Job drawing, mm, ordinate dimensions from the low corner. One solid piece. Give positions to 0.01 mm unless a question says otherwise; leave off trailing zeros. Order: outer loops, then holes, each group sorted by start corner. A loop starts at its lowest first (then second) coordinate and runs counter-clockwise, first axis right, second up.
Item 1: Band-saw the part on B-B on x = 10. Give the cut face in (y, z), plus the area to 3 significant figures.
Item 2: Band-saw the part on C-C on z = 37.5. Give the cut face in (x, y), plus the area to 3 significant figures.
Item 3: Band-saw the part on A-A on y = 2.6. Give the cut face in (x, z).
Item 4: Two-plate mould, pull along Z, no slides. Class the marked faces 1 and 2: released by +Z, released by -Z, zero draft, split by the parting line, or undercut.
Item 5: Wall check: L1, parallel to X at y = 0.3, z = 37.5; L2, parallel to Z at x = 58.5, y = 2.55; L3, parallel to X at y = 2.25, z = 54. Give the ranges that are in metal, low to high.
Item 6: Flat gauge pin, fed straight in: P1, Ø6, axis at x = 16.5, z = 28, coming from the +Y side. Where does the tip first touch, or does it go through?
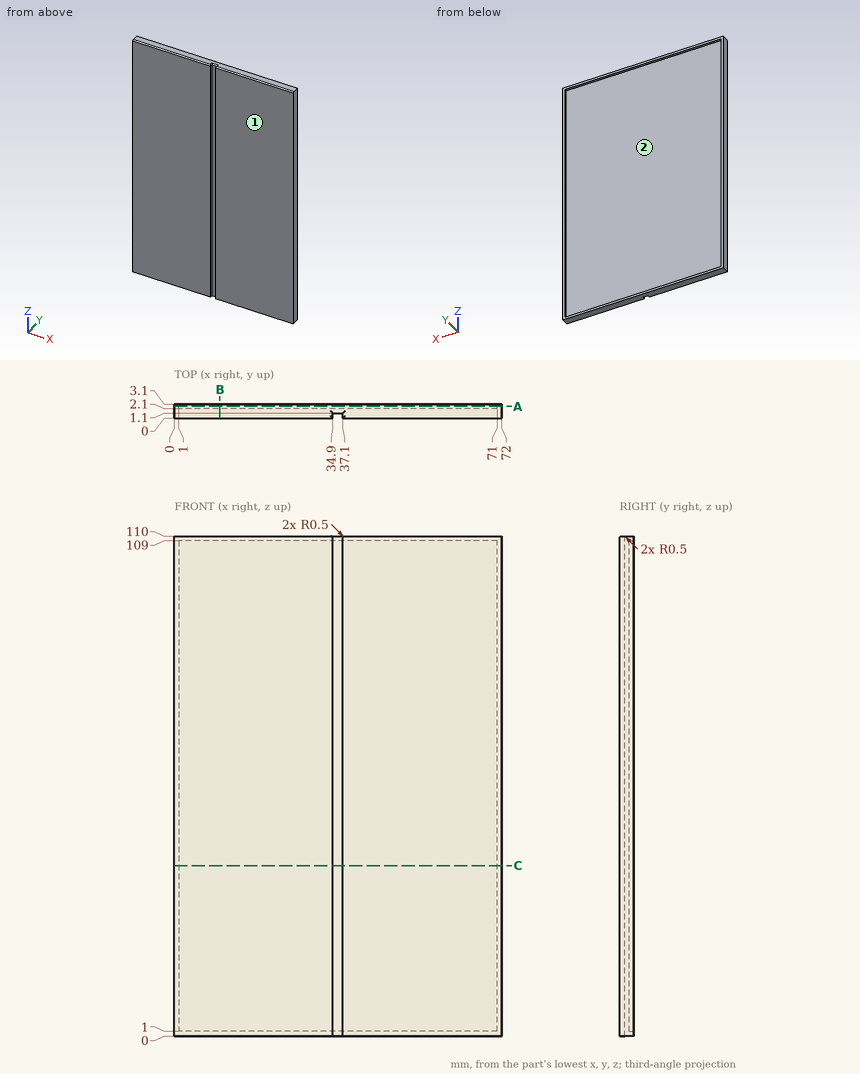
The answers:
1. outline: (0, 0) - (3.1, 0) - (3.1, 1) - (2.1, 1) - (2.1, 109) - (3.1, 109) - (3.1, 110) - (0.5, 110) arc R0.5 ccw to (0, 109.5) - close
1. area: 233 mm2
2. outline: (0, 0) - (34.9, 0) - (34.9, 1.1) - (37.1, 1.1) - (37.1, 0) - (72, 0) - (72, 3.1) - (71, 3.1) - (71, 2.1) - (1, 2.1) - (1, 3.1) - (0, 3.1) - close
2. area: 151 mm2
3. outline: (0, 0) - (72, 0) - (72, 110) - (0, 110) - close; hole (1, 1) - (71, 1) - (71, 109) - (1, 109) - close
4. face 1: zero draft
4. face 2: undercut
5. L1: x = 0 to 34.9, 37.1 to 72
5. L2: z = 0 to 1, 109 to 110
5. L3: x = 0 to 1, 71 to 72
6. P1: stops at y = 2.1
